Could you check a few things on this model? Use its own coordinates, in mm. Face numbers are marked on the shaded views. A direction names the side the tool comes from. Give positions to 0.01 mm unless a question says otherwise; leave off trailing zeros. Order: outer loops, then holes, each group sorted by start corner. A loop starts at its lowest first (then second) coordinate and runs counter-clockwise, first axis right, second up. Notation, with made-up numbers: (77, 6.5) - (88, 6.5) arc R24 ccw to (88, 36.5) - close; hole circle Ø9 at (40.5, 12.25). An arc over 180 degrees is marked (long way). Put each result on its own line as item: value.
Autodesk Inventor part; units mm, degrees
ref_plane "Płaszczyzna konstrukcyjna1" through (-13, 150, -1) normal (0, 0, 1) x (1, 0, 0)
ref_plane "YZ Plane" through (0, 0, 0) normal (1, 0, 0) x (0, 1, 0)
ref_plane "XZ Plane" through (0, 0, 0) normal (0, 1, 0) x (-1, 0, 0)
sketch "Szkic1" plane through (0, 0, 0) normal (0, 1, 0) x (-1, 0, 0)
  circle A0 centre (0, 0) radius 12.5
  circle A1 centre (0, 0) radius 32.5
  dimension "d0" = 25
  dimension "d1" = 65
extrude "Wyciągnięcie proste1" add sketch "Szkic1" along normal blind 150 contours A0 | A1
sketch "Szkic2" plane through (0, 0, 0) normal (0, -1, 0) x (1, 0, 0)
  point P0 (0, 0)
extrude "Wyciągnięcie proste2" cut sketch "Szkic1" along normal blind 100 contours A0
sketch "Szkic3" plane through (0, 150, 0) normal (0, 1, 0) x (1, 0, 0)
  line L0 (13, -13) -> (-13, -13)
  line L1 (-13, -13) -> (-13, 13)
  line L2 (-13, 13) -> (13, 13)
  line L3 (13, 13) -> (13, -13)
  line L4 (13, -13) -> (-13, 13) construction
  line L5 (-13, -13) -> (13, 13) construction
  point P0 (0, 0)
  dimension "d6" = 26
  dimension "d7" = 26
extrude "Wyciągnięcie proste3" add sketch "Szkic3" along normal blind 30
chamfer "Faza1" distance 10 angle 45 2 edges at (0, 180, -13) (0, 180, 13)
sketch "Szkic4" plane through (-13, 180, 3) normal (0, 0.7071, 0.7071) x (1, 0, 0)
  line L0 (26, 0) -> (0, 0)
  line L1 (6, -14) -> (20, -14)
  line L2 (20, -14) -> (20, 0)
  line L3 (20, 0) -> (6, 0)
  line L4 (6, 0) -> (6, -14)
  line L5 (6, -14) -> (20, 0) construction
  line L6 (20, -14) -> (6, 0) construction
  line L7 (0, 0) -> (0, -14.1421)
  point P0 (13, -125.1579)
  point P1 (13, -7)
  dimension "d13" = 14
  dimension "d14" = 14
  dimension "d15" = 6
extrude "Wyciągnięcie proste4" add sketch "Szkic4" along normal blind 30
chamfer "Faza2" distance 14 angle 45 1 edges at (0, 201.2132, 24.2132)
sketch "Szkic5" plane through (-7, 191.3137, 34.1127) normal (0, 1, 0) x (1, 0, 0)
  line L0 (0, 31.1127) -> (0, 19.799)
  line L1 (14, 0) -> (0, 0)
  line L2 (0, 0) -> (0, 19.799)
  line L3 (0, 19.799) -> (14, 19.799)
  line L4 (14, 19.799) -> (14, 0)
  point P0 (7, 34.1127)
  dimension "d21" = 14
  dimension "d22" = 19.799
extrude "Wyciągnięcie proste5" add sketch "Szkic5" along normal blind 30
ref_plane "Płaszczyzna konstrukcyjna1" through (-13, 150, -1) normal (0, 0, 1) x (1, 0, 0)
mirror "Odbij1" about plane through (-13, 150, -1) normal (0, 0, 1) of "Wyciągnięcie proste5", "Wyciągnięcie proste4", "Wyciągnięcie proste3"
equation "\"PromieńGięcia\" = Grubość"
equation "\"SzerokośćGięciaPodcięcia\" = Grubość"
equation "\"GłębokośćGięciaPodcięcia\" = 0.5 * Grubość"
equation "\"RozmiarPodcięciaNarożnika\" = 4 * Grubość"
equation "\"MinimalnaPozostałość\" = 2 * Grubość"
equation "\"PromieńPrzejścia\" = PromieńGięcia"
equation "\"Rozmiar_promienia_Jacobiego\" = PromieńGięcia"
equation "\"Wielk_odstępu\" = Grubość"
properties part number "czesc5"
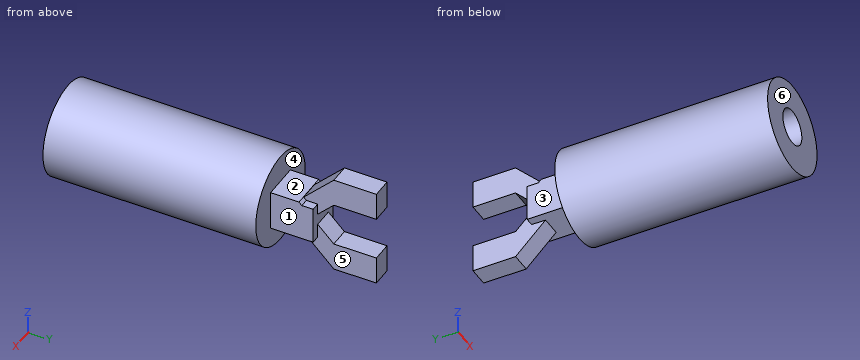
1) Suppose I cut it at A-A, the plane x = 0. List the corners of the cut face in (y, z) for me, and give its area (3 significant figures).
Filled in:
outline: (0, -32.5) - (150, -32.5) - (150, -15) - (170.2, -15) - (191.31, -36.11) - (221.31, -36.11) - (221.31, -16.31) - (191.31, -16.31) - (180, -5) - (180, 3) - (191.31, 14.31) - (221.31, 14.31) - (221.31, 34.11) - (191.31, 34.11) - (170.1, 12.9) - (170, 13) - (150, 13) - (150, 32.5) - (0, 32.5) - (0, 12.5) - (100, 12.5) - (100, -12.5) - (0, -12.5) - close
area: 9,820 mm^2
2) I'm going to push flat-ended pins straight in: pin 1 (10 mm diameter, centred on y = 72.5, z = -15.5, fed in from -X); pin 2 (8 mm diameter, centred on x = -21, y = 61, fed in from +Z); pin 3 (20 mm diameter, centred on x = 0, z = 0, fed in from -Y). Where does each tip first touch, or does it pass through?
Filled in:
pin 1: stops at x = -30.76
pin 2: stops at z = 27.7
pin 3: stops at y = 100
3) Suppose I cut it at D-D, the plane y = 142. List the corners of the cut face in (x, z) for me.
Filled in:
outline: circle Ø65 at (0, 0)
4) If I drill on line 1 (Z direction, x = 0, y = 31.5); line 2 (Y direction, x = 16.5, z = -21.5); line 3 (Z direction, x = 9, y = 80.5), over which ranges is the centre line in solid material (lowest first)? Write a range as [from, to].
Filled in:
line 1: z = [-32.5, -12.5], [12.5, 32.5]
line 2: y = [0, 150]
line 3: z = [-31.23, -8.67], [8.67, 31.23]
5) Which directions (+Z, -Z, +X, -X, +Y, -Y) give clear straight access to the entire face, cutting with the end or side of a thin tool? Please do the marked faces 1, 2 and 3.
Filled in:
face 1: +Z, -Z, +X, +Y
face 2: +Z, +X, -X
face 3: +Z, -Z, -X, +Y
6) We'd pull the mould along Y, two halves only. Please class the marked faces 4, 5 and 6: pulls with the +Y half, pulls with the -Y half, needs draft (parallel to the pull), parting line crosses it, or undercut.
Filled in:
face 4: undercut
face 5: needs draft
face 6: pulls with the -Y half
7) Suppose I cut it at B-B, the plane z = 0. List the corners of the cut face in (x, y) for me.
Filled in:
outline: (-32.5, 0) - (-12.5, 0) - (-12.5, 100) - (12.5, 100) - (12.5, 0) - (32.5, 0) - (32.5, 150) - (13, 150) - (13, 180) - (-13, 180) - (-13, 150) - (-32.5, 150) - close
8) Suppose I cut it at C-C, the plane y = 45.5. List the corners of the cut face in (x, z) for me, and give its area (3 significant figures).
Filled in:
outline: circle Ø65 at (0, 0); hole circle Ø25 at (0, 0)
area: 2,830 mm^2
